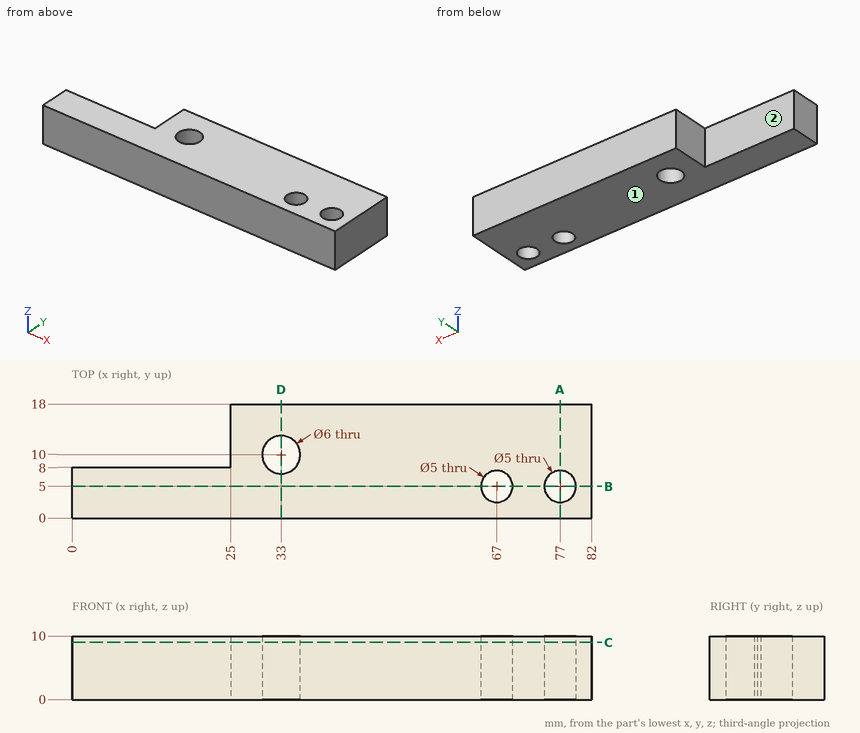
Geometry: see drawing. Coordinates: mm, zero at the bounding-box minimum. A direction names the side the tool comes from. Coordinates: 2 decimals unless noted, no trailing zeros. Order: outer loops, then holes, each group sorted by start corner. A loop starts at its lowest first (then second) coordinate and runs counter-clockwise, first axis right, second up. Notation, with made-up numbers: (38.5, 3.5) - (87.5, 3.5) arc R26 ccw to (87.5, 31.5) - close; hole circle Ø10 at (85, -32). An arc over 180 degrees is marked (long way). Use one line per item in the form item = value.
1) Set-up query: the marked faces 1 and 2. Return all of +Z, -Z, +X, -X, +Y, -Y with unobstructed straight access to the full face (end or side cutting, diameter ignored); none if empty.
Solutions:
face_1 = -Z, +X, -X, +Y, -Y
face_2 = +Z, -Z, -X, +Y
2) Section A-A (x = 77). Return loops of the section in (y, z), then the cut area to 3 significant figures.
Solutions:
outline = (0, 0) - (2.5, 0) - (2.5, 10) - (0, 10) - close; (7.5, 0) - (18, 0) - (18, 10) - (7.5, 10) - close
area = 130 mm^2
3) Ray query, L1, parallel to X at y = 5.25, z = 1.5; L2, parallel to Y at x = 77, z = 7.5; L3, parallel to X at y = 4.5, z = 6. Return the intervals inside material, ascending.
Solutions:
L1 = 0 to 64.51, 69.49 to 74.51, 79.49 to 82
L2 = 0 to 2.5, 7.5 to 18
L3 = 0 to 64.55, 69.45 to 74.55, 79.45 to 82
4) Section D-D (x = 33). Return loops of the section in (y, z), then the cut area to 3 significant figures.
Solutions:
outline = (0, 0) - (7, 0) - (7, 10) - (0, 10) - close; (13, 0) - (18, 0) - (18, 10) - (13, 10) - close
area = 120 mm^2
5) Section C-C (z = 9). Return loops of the section in (x, y).
Solutions:
outline = (0, 0) - (82, 0) - (82, 18) - (25, 18) - (25, 8) - (0, 8) - close; hole circle Ø6 at (33, 10); hole circle Ø5 at (67, 5); hole circle Ø5 at (77, 5)
6) Section B-B (y = 5). Return loops of the section in (x, z), then the cut area to 3 significant figures.
Solutions:
outline = (0, 0) - (64.5, 0) - (64.5, 10) - (0, 10) - close; (69.5, 0) - (74.5, 0) - (74.5, 10) - (69.5, 10) - close; (79.5, 0) - (82, 0) - (82, 10) - (79.5, 10) - close
area = 720 mm^2
7) Pin query (flat end, axial travel): pin 1 (5 mm diameter, centred on x = 9.5, z = 3, fed in from +Y); pin 2 (2 mm diameter, centred on x = 72.5, y = 14, fed in from -Z); pin 3 (3 mm diameter, centred on y = 11, z = 4, fed in from -X). Return the tip coordinate at first contact, or that it passes through.
Solutions:
pin_1 = 8
pin_2 = 0
pin_3 = 25
